from build123d import *

# Parameters (mm, degrees)
F0_W     = 5.4
F0_H     = 19.6
F0_W_2   = 1.8
F0_H_2   = 16
F1_DEPTH = 8
F2_W     = 15.2
F2_H     = 2
F3_DEPTH = 3
F4_W     = 15.2
F4_H     = 6
F5_DEPTH = 2
F6_W     = 9.064092
F6_H     = 1.8
F7_DEPTH = 8.001


with BuildPart() as f1:
    # F0 (on Top) → F1 (new body)
    with BuildSketch(Plane.XY):
        Rectangle(F0_W, F0_H)
        Rectangle(F0_W_2, F0_H_2, mode=Mode.SUBTRACT)
    extrude(amount=F1_DEPTH)

    # F2 (on face) → F3 (join)
    with BuildSketch(Plane(origin=(-2.7, 0, 0), x_dir=(0, -1, 0), z_dir=(-1, 0, 0))):
        with Locations((0, 4)):
            Rectangle(F2_W, F2_H)
    extrude(amount=F3_DEPTH)

    # F4 (on face) → F5 (join)
    with BuildSketch(Plane(origin=(-5.7, 0, 0), x_dir=(0, -1, 0), z_dir=(-1, 0, 0))):
        with Locations((0, 4.1)):
            Rectangle(F4_W, F4_H)
    extrude(amount=F5_DEPTH)

    # F6 (on face) → F7 (cut, through all)
    with BuildSketch(Plane.XY.offset(8)):
        with Locations((-5.432046, 0)):
            Rectangle(F6_W, F6_H)
    extrude(amount=-F7_DEPTH, mode=Mode.SUBTRACT)


solid = f1.part
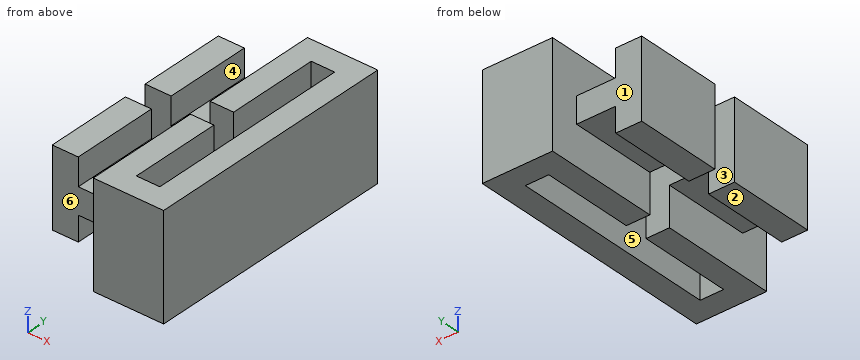
Here's how the part is built. I have some questions about the finished solid (model axes, mm). Face numbers are marked on the shaded views. A direction names the side the tool comes from. Give positions to 0.01 mm unless a question says otherwise; leave off trailing zeros. Order: outer loops, then holes, each group sorted by start corner. A loop starts at its lowest first (then second) coordinate and runs counter-clockwise, first axis right, second up. Notation, with made-up numbers: (64.5, 22.5) -> (109.5, 22.5) arc R17 ccw to (109.5, 55.5) -> close; hole circle Ø11 at (62.25, 17.5). An arc over 180 degrees is marked (long way). Use a Markdown table: item, result. Add a question column.
Item 1: Imagine slicing it at D-D on x = -6.25. Please give me the cut outline in (y, z).
Item 2: Imagine slicing it at A-A on x = -4. Please give me the cut outline in (y, z).
Item 3: If we mould it in two halves opening along Y, with no side actions, what happens to the marked faces 1, 2 and 3? For each: pulls with the +Y half, pulls with the -Y half, needs draft (parallel to the pull), parting line crosses it, or undercut.
Item 4: I need wall thicknesses on line 1 (X direction, y = 1.25, z = 6); line 2 (X direction, y = 5.25, z = 7.5); line 3 (Y direction, x = -2.5, z = 5.5). Which ranges of each line are inside material? Lowest first, please.
Item 5: Imagine slicing it at B-B on y = -2. Please give me the cut outline in (x, z).
Item 6: Will these pins go through, and if not, where does the flat tip stop? pin 1 (3.5 mm diameter, centred on x = -4.5, y = -5, fed in from +Z); pin 2 (2 mm diameter, centred on x = -7, y = -4.5, fed in from -Z).
Item 7: For the marked faces 4, 5 and 6, which set-ups out of +Z, -Z, +X, -X, +Y, -Y let a thin tool reach every point of the face, with its end or its side?
Item 8: Imagine slicing it at C-C on z = 1.75. Please give me the cut outline in (x, y), plus the area to 3 significant figures.
Data:
| question | item | result |
|---|---|---|
| 1 | outline | (-7.6, 1.1) -> (-0.9, 1.1) -> (-0.9, 7.1) -> (-7.6, 7.1) -> close; (0.9, 1.1) -> (7.6, 1.1) -> (7.6, 7.1) -> (0.9, 7.1) -> close |
| 2 | outline | (-7.6, 3) -> (-0.9, 3) -> (-0.9, 5) -> (-7.6, 5) -> close; (0.9, 3) -> (7.6, 3) -> (7.6, 5) -> (0.9, 5) -> close |
| 3 | face 1 | pulls with the +Y half |
| 3 | face 2 | needs draft |
| 3 | face 3 | undercut |
| 4 | line 1 | x = -7.7 to -5.7, -2.7 to -0.9, 0.9 to 2.7 |
| 4 | line 2 | x = -2.7 to -0.9, 0.9 to 2.7 |
| 4 | line 3 | y = -9.8 to -0.9, 0.9 to 9.8 |
| 5 | outline | (-7.7, 1.1) -> (-5.7, 1.1) -> (-5.7, 3) -> (-2.7, 3) -> (-2.7, 0) -> (-0.9, 0) -> (-0.9, 8) -> (-2.7, 8) -> (-2.7, 5) -> (-5.7, 5) -> (-5.7, 7.1) -> (-7.7, 7.1) -> close; (0.9, 0) -> (2.7, 0) -> (2.7, 8) -> (0.9, 8) -> close |
| 6 | pin 1 | stops at z = 7.1 |
| 6 | pin 2 | stops at z = 1.1 |
| 7 | face 4 | +Z, +Y, -Y |
| 7 | face 5 | +Z, -Z |
| 7 | face 6 | +Z, -Z, -X, -Y |
| 8 | outline | (-7.7, -7.6) -> (-5.7, -7.6) -> (-5.7, -0.9) -> (-7.7, -0.9) -> close; (-7.7, 0.9) -> (-5.7, 0.9) -> (-5.7, 7.6) -> (-7.7, 7.6) -> close; (-2.7, -9.8) -> (2.7, -9.8) -> (2.7, 9.8) -> (-2.7, 9.8) -> (-2.7, 0.9) -> (-0.9, 0.9) -> (-0.9, 8) -> (0.9, 8) -> (0.9, -8) -> (-0.9, -8) -> (-0.9, -0.9) -> (-2.7, -0.9) -> close |
| 8 | area | 101 mm² |
